Could you check a few things on this model? Use its own coordinates, in mm. A direction names the side the tool comes from. Give positions to 0.01 mm unless a question says otherwise; leave off trailing zeros. Loops run counter-clockwise (first coordinate to the right, second up) from the corner with the lowest first, then second, coordinate; pieces in that order, holes last. Notation, with made-up numbers: M 50.25,86.5 L 81.25,86.5 A32 cw 81.25,122.5 Z; hole C 35,18.5 d11. An arc over 180 degrees is marked long. Use a Markdown table: item, result. Add a question column.
1) We'd pull the mould along Z, two halves only. Please class faces 1 (the cylindrical face through (-42.952, 2.603, 11.172)), 2 (the flat face through (0, 3, 127)), 3 (the cylindrical face through (22.129, 1.64, 109.865)), 4 (the flat face through (0, 46.635, 63)): +Z half, -Z half, draft (parallel to the pull), parting line (faces both ways), or undercut.
2) Suppose I cut it at C-C on z = 97. List the corners of the cut face in (x, y) for me.
3) Which directions (+Z, -Z, +X, -X, +Y, -Y) give clear straight access to the entire face, cutting with the end or side of a thin tool? Please do faces 5 (the flat face through (-16, 33.935, 63)), 6 (the flat face through (-44.4, -38, 63)).
4) Suppose I cut it at D-D on x = 11.5. List the corners of the cut face in (y, z) for me, and give its area (3 significant figures).
5) Will these pins go through, and if not, where does the flat tip stop? pin 1 Ø6.5 at (y, z) = (2, 59) entering from -X; pin 2 Ø1 at (y, z) = (-10.5, 34.5) entering from -X; pin 3 Ø1 at (y, z) = (-30, 89) entering from -X.
6) If I drill on line 1 along Y through (x, z) = (-19.5, 80); line 2 along Z through (x, y) = (-20, -29); line 3 along Z through (x, y) = (17, -18), over which ranges is the centre line in solid material (lowest first)? Write a range as [from, to].
7) Suppose I cut it at A-A on y = 3. List the corners of the cut face in (x, z) for me, and give its area (3 significant figures).
8) Suppose I cut it at B-B on x = -30. List the corners of the cut face in (y, z) for me, and give its area (3 significant figures).
```python
from build123d import *

# Parameters (mm, degrees)
F0_W     = 90.2906134725
F0_H     = 89.0986584127
F1_DEPTH = 127
F2_T     = -12.7
F3_R     = 5.08
F4_R     = 25.4


with BuildPart() as f1:
    # F0 (on Top) → F1 (new body)
    with BuildSketch(Plane.XY):
        with Locations((0.744972378, 2.0859222859)):
            Rectangle(F0_W, F0_H)
    extrude(amount=F1_DEPTH)

    # F2
    f2_openings = [f1.faces().sort_by_distance(p)[0] for p in [
        (-44.400334, 2.085922, 63.5),
    ]]
    offset(amount=F2_T, openings=f2_openings)

    # F3
    f3_edges = [f1.edges().sort_by_distance(p)[0] for p in [
        (-44.400334, -29.763407, 63.5),
        (-44.400334, 2.085922, 12.7),
        (-44.400334, 33.935251, 63.5),
        (-44.400334, 2.085922, 114.3),
    ]]
    fillet(f3_edges, radius=F3_R)

    # F4
    f4_edges = [f1.edges().sort_by_distance(p)[0] for p in [
        (33.190279, 2.085922, 12.7),
        (33.190279, 33.935251, 63.5),
        (33.190279, 2.085922, 114.3),
        (33.190279, -29.763407, 63.5),
    ]]
    fillet(f4_edges, radius=F4_R)


solid = f1.part
```
Answer block:
| question | item | result |
|---|---|---|
| 1 | face 1 | undercut |
| 1 | face 2 | +Z half |
| 1 | face 3 | undercut |
| 1 | face 4 | draft |
| 2 | outline | M -44.4,-42.46 L 45.89,-42.46 L 45.89,46.64 L -44.4,46.64 L -44.4,39.02 A5.08 ccw -39.32,33.94 L 7.79,33.94 A25.4 cw 31.86,16.64 L 31.86,-12.46 A25.4 cw 7.79,-29.76 L -39.32,-29.76 A5.08 ccw -44.4,-34.84 Z |
| 3 | face 5 | -X |
| 3 | face 6 | +Z, -Z, -X, +Y, -Y |
| 4 | outline | M -42.46,0 L 46.64,0 L 46.64,127 L -42.46,127 Z; hole M -29.49,12.97 L 33.66,12.97 L 33.66,114.03 L -29.49,114.03 Z |
| 4 | area | 4,930 mm^2 |
| 5 | pin 1 | stops at x = 33.19 |
| 5 | pin 2 | stops at x = 32.31 |
| 5 | pin 3 | stops at x = -41.95 |
| 6 | line 1 | y = [-42.46, -29.76], [33.94, 46.64] |
| 6 | line 2 | z = [0, 12.7], [114.3, 127] |
| 6 | line 3 | z = [0, 14.43], [112.57, 127] |
| 7 | outline | M -44.4,0 L 45.89,0 L 45.89,127 L -44.4,127 L -44.4,119.38 A5.08 ccw -39.32,114.3 L 7.79,114.3 A25.4 cw 33.19,88.9 L 33.19,38.1 A25.4 cw 7.79,12.7 L -39.32,12.7 A5.08 ccw -44.4,7.62 Z |
| 7 | area | 3,850 mm^2 |
| 8 | outline | M -42.46,0 L 46.64,0 L 46.64,127 L -42.46,127 Z; hole M -29.76,12.7 L 33.94,12.7 L 33.94,114.3 L -29.76,114.3 Z |
| 8 | area | 4,840 mm^2 |
